Part print with two shaded views. Sizes in mm from the minimum x, y, z corner. Round coordinates to 2 decimals unless told otherwise and drop trailing zeros. Write each loop counter-clockwise with the first axis right and the second up, starting at its lowest first coordinate (ties: lowest second). Pieces come first, ordered by that corner, then holes. Notation, with made-up numbers: M 77,58 L 124,58 A21 cw 124,86 Z; hole C 66,-12 d2. An arc over 180 degrees is marked long. Use one line per item in the form item = value. Start each with the question number.
Item 1: Probe L1, parallel to Z at x = 11.5, y = 5.5; L2, parallel to X at y = 0.7, z = 6; L3, parallel to X at y = 1.15, z = 79. List the from-to ranges inside material, lowest first.
Item 2: Cut at B-B, the plane z = 63.5. Give the cut face in (x, y), then the cut area to 3 significant figures.
Item 3: Cut at C-C, the plane z = 87.5. Give the cut face in (x, y), then the cut area to 3 significant figures.
Item 4: Flat gauge pins, fed straight in: pin 1 Ø1.8 at (y, z) = (3, 21.5) entering from -X; pin 2 Ø0.8 at (y, z) = (3, 91) entering from +X; pin 3 Ø3 at (y, z) = (2, 10) entering from +X; pin 4 Ø0.9 at (x, y) = (73, 2.5) entering from -Z. Where does each tip first touch, or does it go through?
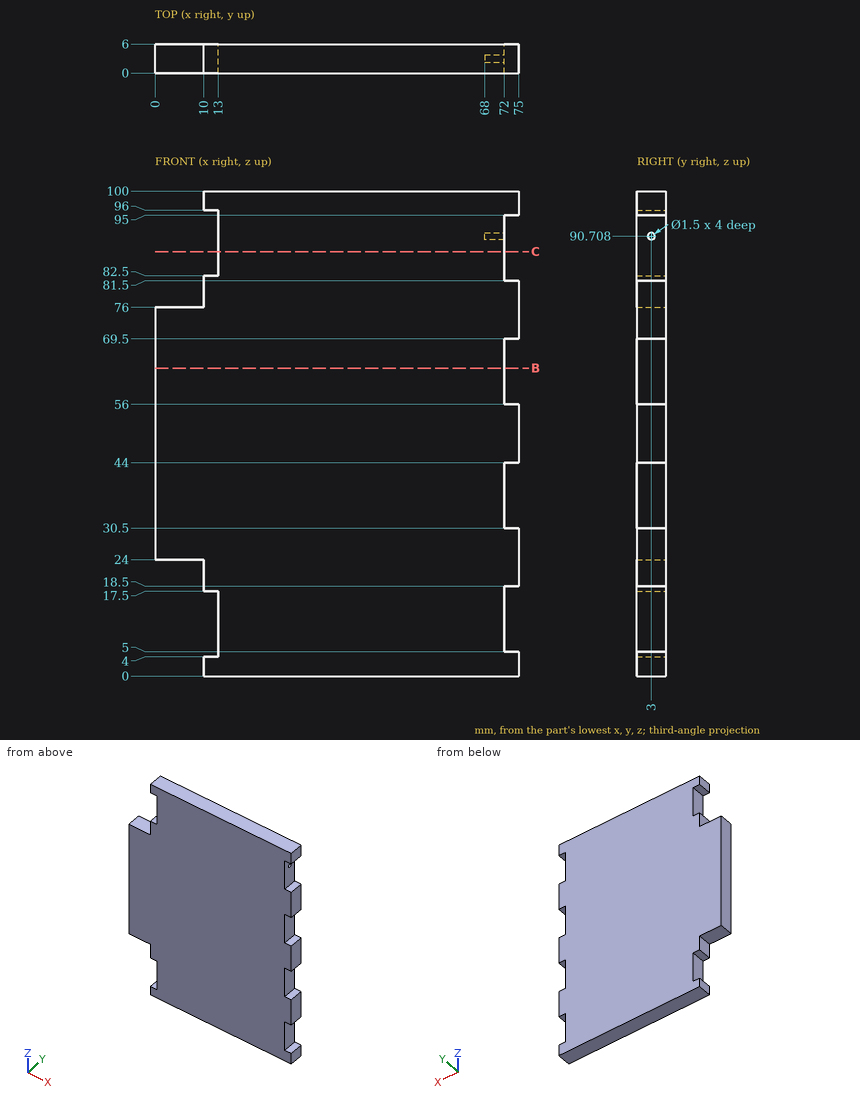
Model answer:
q1.L1 = 0 to 4, 17.5 to 82.5, 96 to 100
q1.L2 = 13 to 72
q1.L3 = 10 to 75
q2.outline = M 0,0 L 72,0 L 72,6 L 0,6 Z
q2.area = 432 mm²
q3.outline = M 13,0 L 72,0 L 72,6 L 13,6 Z
q3.area = 354 mm²
q4.pin_1 = 10
q4.pin_2 = 68
q4.pin_3 = 72
q4.pin_4 = 0
